from build123d import *

# Parameters (mm, degrees)
F0_R     = 1.594655
F1_DEPTH = 5.08
F2_SIZE  = 3.81
F3_R     = 0.635


with BuildPart() as f1:
    # F0 (on Top) → F1 (new body)
    with BuildSketch(Plane.XY):
        with BuildLine():
            Line((4e-06, 50.8), (4.326784, 7.804318))
            ThreePointArc((4.326784, 7.804318), (5.417594, 4.834844), (7.805764, 2.760165))
            ThreePointArc((7.805764, 2.760165), (18.806149, 0.162151), (29.808221, 2.753011))
            ThreePointArc((29.808221, 2.753011), (32.2, 4.829412), (33.291277, 7.802822))
            Line((33.291277, 7.802822), (37.592004, 50.8))
            Line((37.592004, 50.8), (28.067004, 50.8))
            Line((28.067004, 50.8), (28.067004, 41.275))
            Line((28.067004, 41.275), (9.525004, 41.275))
            Line((9.525004, 41.275), (9.525004, 50.8))
            Line((9.525004, 50.8), (4e-06, 50.8))
        make_face()
        with Locations((18.796004, 9.68716)):
            Circle(F0_R, mode=Mode.SUBTRACT)
        with Locations((10.668004, 31.91216)):
            Circle(F0_R, mode=Mode.SUBTRACT)
        with Locations((25.851231, 31.91216)):
            Circle(F0_R, mode=Mode.SUBTRACT)
    extrude(amount=F1_DEPTH)

    # F2
    f2_edges = [f1.edges().sort_by_distance(p)[0] for p in [
        (9.073348, 31.91216, 5.08),
        (24.256576, 31.91216, 5.08),
        (17.201348, 9.68716, 5.08),
    ]]
    chamfer(f2_edges, length=F2_SIZE)

    # F3
    f3_edges = [f1.edges().sort_by_distance(p)[0] for p in [
        (18.806149, 0.162151, 5.08),
        (32.2, 4.829412, 5.08),
        (32.829504, 50.8, 5.08),
        (9.525004, 46.0375, 5.08),
        (35.441641, 29.301411, 5.08),
        (2.163394, 29.302159, 5.08),
        (4.762504, 50.8, 5.08),
        (28.067004, 46.0375, 5.08),
        (5.417594, 4.834844, 5.08),
        (18.796004, 41.275, 5.08),
    ]]
    fillet(f3_edges, radius=F3_R)


solid = f1.part
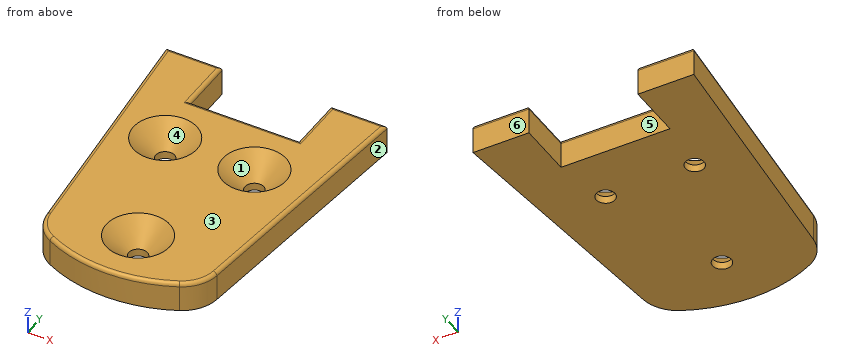
Input: part model. Units: mm. Frame: model coordinates. Face numbers are marked on the shaded views. A direction names the side the tool comes from. Give positions to 0.01 mm unless a question says otherwise; leave off trailing zeros. Loops run counter-clockwise (first coordinate to the right, second up) from the corner with the lowest first, then second, coordinate; pieces in that order, holes last. Notation, with made-up numbers: (22, 82.25) - (58, 82.25) arc R28 cw to (58, 114.25) - close; hole circle Ø2 at (2, 33). An arc over 180 degrees is marked (long way). Use CSV: the item, a comma, the result in double quotes. Start each with the question number.
Item 1: Line query: line 1 (X direction, y = 32.5, z = 3.05); line 2 (X direction, y = 32, z = 2.45); line 3 (Y direction, x = 19.5, z = 4) (3 decimals). Output: solid intervals per line, ascending.
Item 2: Mould query, pull axis Y, two halves, no side actions, for the marked faces 1, 2, 3 and 4. Classes: pulls with the +Y half, pulls with the -Y half, needs draft (parallel to the pull), parting line crosses it, or undercut.
Item 3: Reachability of the marked faces 5 and 6 from +Z, -Z, +X, -X, +Y, -Y: full face, straight path, thin tool, end or side. Return the list, or none.
Item 4: Contact query for flat-ended pins moving along their axis: P1, Ø3, axis at x = 18.8, y = 9.69, coming from the -Z side; P2, Ø3, axis at y = 7.5, z = 2.5, coming from the -X side; P3, Ø1, axis at y = 31.5, z = 4.5, coming from the +X side; P4, Ø1.3, axis at y = 48, z = 2.5, coming from the -X side. Output: stop coordinate, or through.
Item 5: Section A-A on z = 2. Return loops of the section in (x, y) (3 decimals).
Ans:
1,line 1,"x = 1.84 to 7.34, 13.99 to 22.53, 29.17 to 35.76"
1,line 2,"x = 1.89 to 7.89, 13.44 to 23.08, 28.62 to 35.71"
1,line 3,"y = 0.172 to 5.42, 13.954 to 41.275"
2,face 1,"undercut"
2,face 2,"pulls with the -Y half"
2,face 3,"needs draft"
2,face 4,"undercut"
3,face 5,"+Z, -Z, +Y"
3,face 6,"+Z, -Z, +X, -X, +Y"
4,P1,"passes through"
4,P2,"stops at x = 4.21"
4,P3,"stops at x = 35.71"
4,P4,"stops at x = 0.22"
5,outline,"(0, 50.8) - (4.327, 7.804) arc R6.35 ccw to (7.806, 2.76) arc R24.622 ccw to (29.808, 2.753) arc R6.35 ccw to (33.291, 7.803) - (37.592, 50.8) - (28.067, 50.8) - (28.067, 41.275) - (9.525, 41.275) - (9.525, 50.8) - close; hole circle Ø4.649 at (10.668, 31.912); hole circle Ø4.649 at (18.796, 9.687); hole circle Ø4.649 at (25.851, 31.912)"
